Input: part model. Units: mm. Frame: model coordinates. A direction names the side the tool comes from. Round coordinates to 2 decimals unless told otherwise and drop trailing zeros. Loops run counter-clockwise (first coordinate to the right, second up) from the corner with the lowest first, then second, coordinate; pieces in that order, holes last. Notation, with made-up numbers: (19.25, -23) -> (75.25, -23) arc R12 cw to (75.25, -5) -> close; hole circle Ø10 at (52, 36.25). An arc over 180 degrees is marked (long way). Answer as a JSON object with one key per item and string values.
```python
from build123d import *

# Parameters (mm, degrees)
SALIENTE_EXTRUIR1_DEPTH = 25
CROQUIS2_R              = 2.95
SALIENTE_EXTRUIR2_DEPTH = 1.2
CORTAR_EXTRUIR1_DEPTH   = 5.3
SALIENTE_EXTRUIR3_DEPTH = 2.4
CORTAR_EXTRUIR2_DEPTH   = 2.5
CROQUIS6_R              = 1.256804149
SALIENTE_EXTRUIR4_DEPTH = 1.1
CROQUIS7_R              = 1.257398905
SALIENTE_EXTRUIR5_DEPTH = 38


with BuildPart() as part:
    # Croquis1 → Saliente-Extruir1 (new body)
    with BuildSketch(Plane.XY):
        with BuildLine():
            Line((6.443601477, 7.45), (0, 7.45))
            Line((0, 7.45), (-6.443601477, 7.45))
            ThreePointArc((-6.443601477, 7.45), (-9.85, 0), (-6.443601477, -7.45))
            Line((-6.443601477, -7.45), (0, -7.45))
            Line((0, -7.45), (6.443601477, -7.45))
            ThreePointArc((6.443601477, -7.45), (9.85, 0), (6.443601477, 7.45))
        make_face()
    extrude(amount=SALIENTE_EXTRUIR1_DEPTH)

    # Croquis2 → Saliente-Extruir2 (add)
    with BuildSketch(Plane.XY.offset(25)):
        Circle(CROQUIS2_R)
    extrude(amount=SALIENTE_EXTRUIR2_DEPTH)

    # Croquis3 → Cortar-Extruir1 (cut)
    with BuildSketch(Plane(origin=(0, 0, 0), x_dir=(-1, 0, 0), z_dir=(0, 0, -1))):
        with BuildLine():
            Line((-8.2, 1.65), (-9.710818709, 1.65))
            ThreePointArc((-9.710818709, 1.65), (-9.85, 0), (-9.710818709, -1.65))
            Line((-9.710818709, -1.65), (-8.2, -1.65))
            ThreePointArc((-8.2, -1.65), (-6.55, 0), (-8.2, 1.65))
        make_face()
        with BuildLine():
            Line((9.710818709, 1.65), (8.2, 1.65))
            ThreePointArc((8.2, 1.65), (6.55, 0), (8.2, -1.65))
            Line((8.2, -1.65), (9.710818709, -1.65))
            ThreePointArc((9.710818709, -1.65), (9.85, 0), (9.710818709, 1.65))
        make_face()
    extrude(amount=-CORTAR_EXTRUIR1_DEPTH, mode=Mode.SUBTRACT)

    # Croquis4 → Saliente-Extruir3 (add)
    with BuildSketch(Plane(origin=(0, 0, 0), x_dir=(-1, 0, 0), z_dir=(0, 0, -1))):
        with BuildLine():
            Line((3.874274126, 3), (0, 3))
            Line((0, 3), (-3.874274126, 3))
            ThreePointArc((-3.874274126, 3), (0, -4.9), (3.874274126, 3))
        make_face()
    extrude(amount=SALIENTE_EXTRUIR3_DEPTH)

    # Croquis5 → Cortar-Extruir2 (cut)
    with BuildSketch(Plane(origin=(0, 0, -2.4), x_dir=(-1, 0, 0), z_dir=(0, 0, -1))):
        Polygon((0, -3), (-3, -3), (-3, -1.8), (3, -1.8), (3, -3), align=None)
    extrude(amount=-CORTAR_EXTRUIR2_DEPTH, mode=Mode.SUBTRACT)



with BuildPart() as body_2:
    # Croquis6 → Saliente-Extruir4 (new body)
    with BuildSketch(Plane(origin=(0, 0, -2.4), x_dir=(-1, 0, 0), z_dir=(0, 0, -1))):
        Circle(CROQUIS6_R)
    extrude(amount=SALIENTE_EXTRUIR4_DEPTH)


with BuildPart() as part_1:
    add(part.part)

    add(body_2.part)  # Saliente-Extruir5 merges body 2
    # Croquis7 → Saliente-Extruir5 (add)
    with BuildSketch(Plane(origin=(0, 0, -3.5), x_dir=(-1, 0, 0), z_dir=(0, 0, -1))):
        Circle(CROQUIS7_R)
    extrude(amount=-SALIENTE_EXTRUIR5_DEPTH)


solid = part_1.part
```
1) Section D-D, the plane z = 24. Output: boundary loops of the cut face in (x, y), plus the area to 3 significant figures.
Output:
{"outline": "(-6.44, -7.45) -> (6.44, -7.45) arc R9.85 ccw to (6.44, 7.45) -> (-6.44, 7.45) arc R9.85 ccw to start", "area": "262 mm^2"}
2) Reachability of faces 1 (the face through (1, -1, 26.2)), 2 (the face through (0, 3, -1)), 3 (the face through (-0.1, 3.4, 0)), 4 (the face through (-8, 0, 5.3)) from +Z, -Z, +X, -X, +Y, -Y: full face, straight path, thin tool, end or side. Return the list, or none.
Output:
{"face 1": "+Z", "face 2": "-Z, +X, -X, +Y", "face 3": "-Z", "face 4": "-Z, -X"}
3) Ray query, probe 1 along Z at (x, y) = (-1.75, 6); probe 2 along Z at (x, y) = (4.5, 0.5); probe 3 along X at (y, z) = (0, 3.5). Return the intervals inside material, ascending.
Output:
{"probe 1": "z = 0 to 25", "probe 2": "z = -2.4 to 25", "probe 3": "x = -6.55 to 6.55"}
4) Section A-A, the plane x = 0. Output: boundary loops of the cut face in (y, z).
Output:
{"outline": "(-7.45, 0) -> (-4.9, 0) -> (-4.9, -2.4) -> (-3, -2.4) -> (-3, 0.1) -> (-1.8, 0.1) -> (-1.8, -2.4) -> (-1.26, -2.4) -> (-1.26, -3.5) -> (1.26, -3.5) -> (1.26, -2.4) -> (3, -2.4) -> (3, 0) -> (7.45, 0) -> (7.45, 25) -> (2.95, 25) -> (2.95, 26.2) -> (1.26, 26.2) -> (1.26, 34.5) -> (-1.26, 34.5) -> (-1.26, 26.2) -> (-2.95, 26.2) -> (-2.95, 25) -> (-7.45, 25) -> close"}
5) Section B-B, the plane z = 4. Output: boundary loops of the cut face in (x, y).
Output:
{"outline": "(-9.71, -1.65) arc R9.85 ccw to (-6.44, -7.45) -> (6.44, -7.45) arc R9.85 ccw to (9.71, -1.65) -> (8.2, -1.65) arc R1.65 cw to (8.2, 1.65) -> (9.71, 1.65) arc R9.85 ccw to (6.44, 7.45) -> (-6.44, 7.45) arc R9.85 ccw to (-9.71, 1.65) -> (-8.2, 1.65) arc R1.65 cw to (-8.2, -1.65) -> close"}
6) Contact query for flat-ended pins moving along their axis: P1, Ø1.2, axis at x = -0.5, z = -1.5, coming from the +Y side; P2, Ø1.2, axis at x = 9, z = 3.5, coming from the +Y side; P3, Ø1, axis at x = -7.5, z = 22, coming from the +Y side. Output: stop coordinate, or through.
Output:
{"P1": "stops at y = 3", "P2": "stops at y = 5.14", "P3": "stops at y = 6.93"}
7) Section C-C, the plane y = 0. Output: boundary loops of the cut face in (x, z).
Output:
{"outline": "(-9.85, 5.3) -> (-6.55, 5.3) -> (-6.55, 0) -> (-4.9, 0) -> (-4.9, -2.4) -> (-1.26, -2.4) -> (-1.26, -3.5) -> (1.26, -3.5) -> (1.26, -2.4) -> (4.9, -2.4) -> (4.9, 0) -> (6.55, 0) -> (6.55, 5.3) -> (9.85, 5.3) -> (9.85, 25) -> (2.95, 25) -> (2.95, 26.2) -> (1.26, 26.2) -> (1.26, 34.5) -> (-1.26, 34.5) -> (-1.26, 26.2) -> (-2.95, 26.2) -> (-2.95, 25) -> (-9.85, 25) -> close"}
8) Draft query along X for faces 5 (the face through (3, -2, -1)), 6 (the face through (0.153, -4.898, -1.183)), 7 (the face through (9.85, -0.12, 12.32)). Return one class per face: +X half, -X half, draft (parallel to the pull), parting line (faces both ways), or undercut.
Output:
{"face 5": "undercut", "face 6": "parting line", "face 7": "+X half"}
